Input: part model. Units: mm. Frame: model coordinates. A direction names the side the tool comes from. Round coordinates to 2 decimals unless told otherwise and drop trailing zeros. Loops run counter-clockwise (first coordinate to the right, second up) from the corner with the lowest first, then second, coordinate; pieces in that order, holes last. Notation, with made-up numbers: (-34.75, 61.25) -> (-30.75, 61.25) arc R35 cw to (-30.75, 98.25) -> close; hole circle Ø10 at (27.25, 80). An arc over 180 degrees is marked (long way). One line per question, with ' | ' between items. Start each with the question number.
Q1. Mould query, pull axis X, two halves, no side actions, for faces 4 (the face through (-16, 16, 28.75)), 5 (the face through (-19.031, -18.976, 16.639)), 6 (the face through (0, 0, 57.75)). Classes: pulls with the +X half, pulls with the -X half, needs draft (parallel to the pull), parting line crosses it, or undercut.
Q2. Material intervals for L1, parallel to Y at x = -15.5, z = 30.7; L2, parallel to Z at x = -8, y = -19; L3, parallel to X at y = 14, z = 7.5, sorted ascending.
Q3. Cut plane D-D on y = -13. Return loops of the section in (x, z).
Q4. Cut plane C-C on z = 24.5. Return loops of the section in (x, y), and give its area (3 significant figures).
Q5. Cut plane A-A on z = 32. Return loops of the section in (x, y), and give its area (3 significant figures).
Q6. Contact query for flat-ended pins moving along their axis: P1, Ø0.9, axis at x = -15.5, y = 15.5, coming from the -Z side; P2, Ø2.5, axis at x = -15.5, y = 15.5, coming from the +Z side; P3, Ø4, axis at x = 15.5, y = -15.5, coming from the +Z side; P4, Ø3, axis at x = -23.5, z = 33.5, coming from the +Y side. Output: stop coordinate, or through.
Q7. Access query for faces 1 (the face through (15, -15, 5)), 2 (the face through (-2.38, -10.74, 34.48)), 3 (the face through (0, -21, 17)). Directions: +Z, -Z, +X, -X, +Y, -Y. A direction counts if a zero-diameter tool reaches every point of the face in a straight line with its end or side. Return the directions, or none.
Q8. Cut plane B-B on x = 0. Return loops of the section in (y, z).
from build123d import *

# Parameters (mm, degrees)
BOSS_EXTRUDE1_DEPTH = 33.75
SKETCH2_R           = 16.5
CUT_EXTRUDE1_DEPTH  = 0.5
SKETCH3_R           = 11
BOSS_EXTRUDE2_DEPTH = 2.5
SKETCH4_R           = 3.5
CUT_EXTRUDE2_DEPTH  = 5
BOSS_EXTRUDE3_DEPTH = 27
SKETCH6_R           = 1.5
CUT_EXTRUDE3_DEPTH  = 5
SKETCH7_W           = 10
SKETCH7_H           = 17
BOSS_EXTRUDE4_DEPTH = 8.7


with BuildPart() as part:
    # Sketch1 → Boss-Extrude1 (new body)
    with BuildSketch(Plane.XY):
        Polygon((-17.006989489, 21), (-21, 17.006989489), (-21, -17.006989489), (-17.006989489, -21), (17.006989489, -21), (21, -17.006989489), (21, 17.006989489), (17.006989489, 21), align=None)
    extrude(amount=BOSS_EXTRUDE1_DEPTH)

    # Sketch2 → Cut-Extrude1 (cut)
    with BuildSketch(Plane.XY.offset(33.75)):
        Circle(SKETCH2_R)
    extrude(amount=-CUT_EXTRUDE1_DEPTH, mode=Mode.SUBTRACT)

    # Sketch3 → Boss-Extrude2 (add)
    with BuildSketch(Plane.XY.offset(33.25)):
        Circle(SKETCH3_R)
    extrude(amount=BOSS_EXTRUDE2_DEPTH)

    # Sketch4 → Cut-Extrude2 (cut)
    with BuildSketch(Plane.XY.offset(35.75)):
        Circle(SKETCH4_R)
    extrude(amount=-CUT_EXTRUDE2_DEPTH, mode=Mode.SUBTRACT)

    # Sketch5 → Boss-Extrude3 (add)
    with BuildSketch(Plane.XY.offset(30.75)):
        with BuildLine():
            Line((-1.5, 2), (1.5, 2))
            ThreePointArc((1.5, 2), (0, -2.5), (-1.5, 2))
        make_face()
    extrude(amount=BOSS_EXTRUDE3_DEPTH)

    # Sketch6 → Cut-Extrude3 (cut)
    with BuildSketch(Plane.XY.offset(33.75)):
        with Locations((-15.5, 15.5)):
            Circle(SKETCH6_R)
        with Locations((15.5, 15.5)):
            Circle(SKETCH6_R)
        with Locations((15.5, -15.5)):
            Circle(SKETCH6_R)
        with Locations((-15.5, -15.5)):
            Circle(SKETCH6_R)
    cut_extrude3 = extrude(amount=-CUT_EXTRUDE3_DEPTH, mode=Mode.SUBTRACT)

    # Mirror1: Cut-Extrude3 across plane
    add(cut_extrude3.mirror(Plane(origin=(0, 0, 16.875), x_dir=(1, 0, 0), z_dir=(0, 0, -1))), mode=Mode.SUBTRACT)

    # Sketch7 → Boss-Extrude4 (add)
    with BuildSketch(Plane.ZY.offset(21)):
        with Locations((5, 0)):
            Rectangle(SKETCH7_W, SKETCH7_H)
    extrude(amount=BOSS_EXTRUDE4_DEPTH)


solid = part.part
Results:
1) face 4: undercut | face 5: pulls with the -X half | face 6: needs draft
2) L1: -21 to -17, -14 to 14, 17 to 21 | L2: 0 to 33.75 | L3: -21 to 21
3) outline: (-21, 0) -> (21, 0) -> (21, 33.75) -> (10.16, 33.75) -> (10.16, 33.25) -> (-10.16, 33.25) -> (-10.16, 33.75) -> (-21, 33.75) -> close
4) outline: (-21, -17.01) -> (-17.01, -21) -> (17.01, -21) -> (21, -17.01) -> (21, 17.01) -> (17.01, 21) -> (-17.01, 21) -> (-21, 17.01) -> close | area: 1,730 mm^2
5) outline: (-21, -17.01) -> (-17.01, -21) -> (17.01, -21) -> (21, -17.01) -> (21, 17.01) -> (17.01, 21) -> (-17.01, 21) -> (-21, 17.01) -> close; (-1.5, 2) arc R2.5 ccw (long way) to (1.5, 2) -> close; hole circle Ø3 at (-15.5, -15.5); hole circle Ø3 at (-15.5, 15.5); hole circle Ø7 at (0, 0); hole circle Ø3 at (15.5, -15.5); hole circle Ø3 at (15.5, 15.5) | area: 1,680 mm^2
6) P1: z = 5 | P2: z = 28.75 | P3: z = 33.75 | P4: through
7) face 1: -Z | face 2: +Z | face 3: +Z, -Z, +X, -X, -Y
8) outline: (-21, 0) -> (21, 0) -> (21, 33.75) -> (16.5, 33.75) -> (16.5, 33.25) -> (11, 33.25) -> (11, 35.75) -> (3.5, 35.75) -> (3.5, 30.75) -> (2, 30.75) -> (2, 57.75) -> (-2.5, 57.75) -> (-2.5, 30.75) -> (-3.5, 30.75) -> (-3.5, 35.75) -> (-11, 35.75) -> (-11, 33.25) -> (-16.5, 33.25) -> (-16.5, 33.75) -> (-21, 33.75) -> close
